The model under review builds one solid part; all positions refer to its coordinate system, in mm. A direction names the side the tool comes from. Round coordinates to 2 decimals unless told otherwise and drop trailing zeros. Order: outer loops, then holes, each group sorted by start corner. A loop starts at its lowest first (then second) coordinate and runs counter-clockwise, first axis right, second up. Notation, with made-up numbers: M 77.5,36.25 L 101.5,36.25 A14 ccw 101.5,49.25 Z; hole C 38,46.25 d5. An arc over 180 degrees is marked long. Answer as a JSON object with one key per item and string values. Group by question number.
1. Add section D-D on z = 15. State the section outline as (x, y) points, and give its area (3 significant figures).
2. Add section C-C on x = -15. State the section outline as (y, z) points, and give its area (3 significant figures).
3. Add section A-A on y = 2.75. State the section outline as (x, z) points.
4. Machinability: for faces 5 (the face through (-13.451, -10, 0)), 6 (the face through (4.5, 9.7, -8.9)), 7 (the face through (-12.9, -9.7, 17.3)), 8 (the face through (-12.9, 9.7, -17.3)), 9 (the face through (19, 10, -13.451)), which of the approach directions +Z, -Z, +X, -X, +Y, -Y give a long, thin tool a straight path to every point of the face, cutting with its end or side? Answer none if there is none.
5. Add section B-B on z = -3.5. State the section outline as (x, y) points.
6. Clearance check with flat-ended pins moving along their axes: P1, Ø3, axis at x = -16.5, y = -7, coming from the -Z side; P2, Ø0.8, axis at y = -10, z = -19, coming from the -X side; P3, Ø1.2, axis at y = 9.5, z = -19.5, coming from the +X side. State where each tip first meets the part, or that it passes through.
7. To check wall thickness, follow probe 1 along Z at (x, y) = (0, -6.5); probe 2 along Y at (x, z) = (7, -5.5). State the ranges of each line that lie inside material, in increasing order. Write a range as [from, to].
8. Mouldability with a two-part tool opening along X and no side actions: class faces 1 (the face through (20.68, -0.15, 14.27)), 2 (the face through (0, 0, -21.15)), 3 (the face through (-13.451, -10, 19)), 4 (the face through (-4.5, -9.7, -8.9)) as released by +X, released by -X, zero draft, split by the parting line, or undercut.
```python
from build123d import *

# Parameters (mm, degrees)
BOSS_EXTRUDE1_DEPTH = 11
SKETCH18_W          = 3.3
SKETCH18_H          = 2.5
CUT_EXTRUDE10_DEPTH = 43.3
SKETCH19_W          = 3.3
SKETCH19_H          = 2.5
CUT_EXTRUDE11_DEPTH = 43.3
SKETCH20_W          = 6.221233688
SKETCH20_H          = 2.5
CUT_EXTRUDE12_DEPTH = 57.710616844
SKETCH21_W          = 6.221233688
SKETCH21_H          = 2.5
CUT_EXTRUDE13_DEPTH = 57.710616844
SKETCH22_R          = 2.5
CUT_EXTRUDE14_DEPTH = 9.5
CUT_EXTRUDE15_DEPTH = 20.5
FILLET8_R           = 6


with BuildPart() as part:
    # Sketch1 → Boss-Extrude1 (new body)
    with BuildSketch(Plane(origin=(0, 0, 0), x_dir=(1, 0, 0), z_dir=(0, 1, 0))):
        Polygon((-21.15, 16.750923472), (-16.750923472, 21.15), (16.750923472, 21.15), (21.15, 16.750923472), (21.15, -16.750923472), (16.750923472, -21.15), (-16.750923472, -21.15), (-21.15, -16.750923472), align=None)
    boss_extrude1 = extrude(amount=BOSS_EXTRUDE1_DEPTH)

    # Sketch18 → Cut-Extrude10 (cut, through all)
    with BuildSketch(Plane.XY.offset(21.15)):
        with Locations((15.100923472, 9.75)):
            Rectangle(SKETCH18_W, SKETCH18_H)
        with Locations((-15.100923472, 9.75)):
            Rectangle(SKETCH18_W, SKETCH18_H)
    cut_extrude10 = extrude(amount=-CUT_EXTRUDE10_DEPTH, mode=Mode.SUBTRACT)

    # Sketch19 → Cut-Extrude11 (cut, through all)
    with BuildSketch(Plane(origin=(21.15, 0, 0), x_dir=(0, 0, -1), z_dir=(1, 0, 0))):
        with Locations((-15.100923472, 9.75)):
            Rectangle(SKETCH19_W, SKETCH19_H)
        with Locations((15.100923472, 9.75)):
            Rectangle(SKETCH19_W, SKETCH19_H)
    cut_extrude11 = extrude(amount=-CUT_EXTRUDE11_DEPTH, mode=Mode.SUBTRACT)

    # Sketch20 → Cut-Extrude12 (cut, through all)
    with BuildSketch(Plane(origin=(18.950461736, 0, 18.950461736), x_dir=(0.707106781, 0, -0.707106781), z_dir=(0.707106781, 0, 0.707106781))):
        with Locations((0, 9.75)):
            Rectangle(SKETCH20_W, SKETCH20_H)
    cut_extrude12 = extrude(amount=-CUT_EXTRUDE12_DEPTH, mode=Mode.SUBTRACT)

    # Sketch21 → Cut-Extrude13 (cut, through all)
    with BuildSketch(Plane(origin=(-18.950461736, 0, 18.950461736), x_dir=(0.707106781, 0, 0.707106781), z_dir=(-0.707106781, 0, 0.707106781))):
        with Locations((0, 9.75)):
            Rectangle(SKETCH21_W, SKETCH21_H)
    cut_extrude13 = extrude(amount=-CUT_EXTRUDE13_DEPTH, mode=Mode.SUBTRACT)

    # Sketch22 → Cut-Extrude14 (cut, through all)
    with BuildSketch(Plane(origin=(0, 8.5, 0), x_dir=(1, 0, 0), z_dir=(0, 1, 0))):
        Circle(SKETCH22_R)
    cut_extrude14 = extrude(amount=-CUT_EXTRUDE14_DEPTH, mode=Mode.SUBTRACT)

    # Mirror1: Boss-Extrude1, Cut-Extrude10, Cut-Extrude11, Cut-Extrude12, Cut-Extrude13, Cut-Extrude14 across plane
    add(boss_extrude1.mirror(Plane(origin=(0, 0, 0), x_dir=(0, 0, 1), z_dir=(0, -1, 0))))
    add(cut_extrude10.mirror(Plane(origin=(0, 0, 0), x_dir=(0, 0, 1), z_dir=(0, -1, 0))), mode=Mode.SUBTRACT)
    add(cut_extrude11.mirror(Plane(origin=(0, 0, 0), x_dir=(0, 0, 1), z_dir=(0, -1, 0))), mode=Mode.SUBTRACT)
    add(cut_extrude12.mirror(Plane(origin=(0, 0, 0), x_dir=(0, 0, 1), z_dir=(0, -1, 0))), mode=Mode.SUBTRACT)
    add(cut_extrude13.mirror(Plane(origin=(0, 0, 0), x_dir=(0, 0, 1), z_dir=(0, -1, 0))), mode=Mode.SUBTRACT)
    add(cut_extrude14.mirror(Plane(origin=(0, 0, 0), x_dir=(0, 0, 1), z_dir=(0, -1, 0))), mode=Mode.SUBTRACT)

    # Sketch23 → Cut-Extrude15 (cut, through all)
    with BuildSketch(Plane(origin=(0, 8.5, 0), x_dir=(1, 0, 0), z_dir=(0, 1, 0))):
        Polygon((-21.15, -14.432485579), (-14.432485579, -21.15), (-16.750923472, -21.15), (-21.15, -16.750923472), align=None)
        Polygon((-21.15, 14.432485579), (-14.432485579, 21.15), (-16.750923472, 21.15), (-21.15, 16.750923472), align=None)
        Polygon((14.432485579, 21.15), (21.15, 14.432485579), (21.15, 16.750923472), (16.750923472, 21.15), align=None)
        Polygon((14.432485579, -21.15), (21.15, -14.432485579), (21.15, -16.750923472), (16.750923472, -21.15), align=None)
    extrude(amount=-CUT_EXTRUDE15_DEPTH, mode=Mode.SUBTRACT)

    # Fillet8
    fillet8_edges = [part.edges().sort_by_distance(p)[0] for p in [
        (14.432485579, 0, -21.15),
        (21.15, 0, -14.432485579),
        (-21.15, 0, -14.432485579),
        (-14.432485579, 0, -21.15),
        (-14.432485579, 0, 21.15),
        (-21.15, 0, 14.432485579),
        (21.15, 0, 14.432485579),
        (14.432485579, 0, 21.15),
    ]]
    fillet(fillet8_edges, radius=FILLET8_R)


solid = part.part
```
Recorded:
{
 "1": {"outline": "M -20.32,-8.5 L 20.32,-8.5 L 20.32,8.5 L -20.32,8.5 Z", "area": "691 mm²"},
 "2": {"outline": "M -8.5,-20.32 L 8.5,-20.32 L 8.5,20.32 L -8.5,20.32 Z", "area": "691 mm²"},
 "3": {"outline": "M -21.15,-11.95 A6 ccw -19.39,-16.19 L -16.19,-19.39 A6 ccw -11.95,-21.15 L 11.95,-21.15 A6 ccw 16.19,-19.39 L 19.39,-16.19 A6 ccw 21.15,-11.95 L 21.15,11.95 A6 ccw 19.39,16.19 L 16.19,19.39 A6 ccw 11.95,21.15 L -11.95,21.15 A6 ccw -16.19,19.39 L -19.39,16.19 A6 ccw -21.15,11.95 Z; hole C 0,0 d5"},
 "4": {"face 5": "+Z, -Z, -Y", "face 6": "+Y", "face 7": "-X, -Y", "face 8": "-X, +Y", "face 9": "-Z, +X, -X, +Y"},
 "5": {"outline": "M -21.15,-11 L -16.75,-11 L -16.75,-8.5 L -13.45,-8.5 L -13.45,-11 L -7.9,-11 L -7.9,-8.5 L 7.9,-8.5 L 7.9,-11 L 13.45,-11 L 13.45,-8.5 L 16.75,-8.5 L 16.75,-11 L 21.15,-11 L 21.15,11 L 16.75,11 L 16.75,8.5 L 13.45,8.5 L 13.45,11 L 7.9,11 L 7.9,8.5 L -7.9,8.5 L -7.9,11 L -13.45,11 L -13.45,8.5 L -16.75,8.5 L -16.75,11 L -21.15,11 Z"},
 "6": {"P1": "stops at z = -20.32", "P2": "stops at x = -13.45", "P3": "stops at x = 13.45"},
 "7": {"probe 1": "z = [-21.15, -2.5], [2.5, 21.15]", "probe 2": "y = [-8.5, 8.5]"},
 "8": {"face 1": "released by +X", "face 2": "zero draft", "face 3": "released by -X", "face 4": "undercut"}
}
